Check sheet for the modelled part. Datum: model origin and axes. Units: mm. A direction names the side the tool comes from. Round coordinates to 2 decimals unless told otherwise and drop trailing zeros. Order: outer loops, then holes, each group sorted by start corner. A loop starts at its lowest first (then second) coordinate and runs counter-clockwise, first axis right, second up.
from build123d import *

# Parameters (mm, degrees)
F1_DEPTH = 50
F2_T     = -4
F3_R     = 5
F5_D     = 20
F6_W     = 4
F6_H     = 60
F7_DEPTH = 42
F9_D     = 40
F9_DEPTH = 4
F9_TIP   = 12.0172123806


with BuildPart() as f1:
    # F0 (on Front) → F1 (new body)
    with BuildSketch(Plane.XZ):
        Polygon((-50, -430), (-30, -500), (30, -500), (50, -430), (50, 500), (-50, 500), align=None)
    extrude(amount=F1_DEPTH)

    # F2
    f2_openings = [f1.faces().sort_by_distance(p)[0] for p in [
        (0, -25, -500),
        (-40, -25, -465),
        (40, -25, -465),
    ]]
    offset(amount=F2_T, openings=f2_openings)

    # F3
    f3_edges = [f1.edges().sort_by_distance(p)[0] for p in [
        (50, -50, 35),
        (50, 0, 35),
        (-50, 0, 35),
        (-50, -50, 35),
        (-46, -4, 26),
        (46, -4, 26),
        (46, -46, 26),
        (-46, -46, 26),
    ]]
    fillet(f3_edges, radius=F3_R)

    # F5 (through all)
    with Locations(Plane(origin=(0, 0, 0), x_dir=(-1, 0, 0), z_dir=(0, 1, 0))):
        with Locations((0, -500)):
            Hole(F5_D / 2)

    # F6 (on face) → F7 (join)
    with BuildSketch(Plane.XZ.offset(4)):
        with Locations((0, -450)):
            Rectangle(F6_W, F6_H)
    extrude(amount=F7_DEPTH)

    # F9 (one way)
    with BuildSketch(Plane(origin=(-2, 0, 0), x_dir=(0, -1, 0), z_dir=(-1, 0, 0))):
        with Locations((25, -480), (25, -420)):
            Circle(F9_D / 2)
    extrude(amount=-F9_DEPTH, mode=Mode.SUBTRACT)
    with Locations(Plane(origin=(-2, 0, 0), x_dir=(0, -1, 0), z_dir=(-1, 0, 0))):
        with Locations((25, -480), (25, -420)):
            with Locations((0, 0, -(F9_DEPTH + F9_TIP / 2))):  # 118° drill point
                Cone(0, F9_D / 2, F9_TIP, mode=Mode.SUBTRACT)


solid = f1.part
1) Gauge pin test, flat ends, axial feed: pin 1 (0.8 mm diameter, centred on x = 0, y = -45.5, fed in from -Z); pin 2 (12.5 mm diameter, centred on y = -31, z = -437.5, fed in from -X). Record the tip position at first contact, or that the pin passes through.
2) Sectioned sample at A-A on y = -25. Record the cut outline in (x, z), and give its area (3 significant figures).
3) Draft check along Y on faces 1 (the face through (-46.8, -24.6, -441.2)), 2 (the face through (-1, 0, 7)), 3 (the face through (0, -25, -440)). Enter one of: pulls with the +Y half, pulls with the -Y half, needs draft (parallel to the pull), parting line crosses it, or undercut.
4) Scan lines: line 1 (Y direction, x = -16, z = 97); line 2 (Y direction, x = -42, z = -43); line 3 (X direction, y = -32, z = 212). Record each from-to range of solid material in increasing order.
5) Sectioned sample at B-B on z = 339. Record the cut outline in (x, y).
6) Set-up check for faces 4 (the face through (0, -25, -460)), 5 (the face through (2, -25, -450)): record each of +Z, -Z, +X, -X, +Y, -Y from which the full face is reachable in a straight line by a thin tool's end or side.
Values found:
1. pin 1: stops at z = -480
1. pin 2: stops at x = -49.64
2. outline: (-50, -430) - (-46, -444) - (-46, 496) - (46, 496) - (46, -444) - (50, -430) - (50, 500) - (-50, 500) - close; (-2, -460) - (2, -460) - (2, -440) - (-2, -440) - close
2. area: 7,940 mm2
3. face 1: needs draft
3. face 2: pulls with the +Y half
3. face 3: undercut
4. line 1: y = -50 to -46, -4 to 0
4. line 2: y = -50 to -45.9, -4.1 to 0
4. line 3: x = -50 to -46, 46 to 50
5. outline: (-50, -45) arc R5 ccw to (-45, -50) - (45, -50) arc R5 ccw to (50, -45) - (50, -5) arc R5 ccw to (45, 0) - (-45, 0) arc R5 ccw to (-50, -5) - close; hole (-46, -41) arc R5 ccw to (-41, -46) - (41, -46) arc R5 ccw to (46, -41) - (46, -9) arc R5 ccw to (41, -4) - (-41, -4) arc R5 ccw to (-46, -9) - close
6. face 4: -Z, +X, -X
6. face 5: -Z
